from build123d import *

# Parameters (mm, degrees)
SKETCH1_W           = 35
SKETCH1_H           = 15
SKETCH1_R           = 5.5
BOSS_EXTRUDE1_DEPTH = 7
SKETCH2_W           = 4
SKETCH2_H           = 15
BOSS_EXTRUDE2_DEPTH = 40


with BuildPart() as part:
    # Sketch1 → Boss-Extrude1 (new body)
    with BuildSketch(Plane.XY):
        Rectangle(SKETCH1_W, SKETCH1_H)
        Circle(SKETCH1_R, mode=Mode.SUBTRACT)
    extrude(amount=BOSS_EXTRUDE1_DEPTH)

    # Sketch2 → Boss-Extrude2 (add)
    with BuildSketch(Plane.XY.offset(7)):
        with Locations((19.5, 0)):
            Rectangle(SKETCH2_W, SKETCH2_H)
        with Locations((-19.5, 0)):
            Rectangle(SKETCH2_W, SKETCH2_H)
    extrude(amount=-BOSS_EXTRUDE2_DEPTH)


solid = part.part
Geometry: final body of the model. Coordinates: model frame, mm. A direction names the side the tool comes from. Round coordinates to 2 decimals unless told otherwise and drop trailing zeros. Write each loop counter-clockwise with the first axis right and the second up, starting at its lowest first coordinate (ties: lowest second). Pieces come first, ordered by that corner, then holes. Notation, with made-up numbers: M 26.5,83 L 54.5,83 A14 ccw 54.5,94 Z; hole C 0.25,65.5 d8. An arc over 180 degrees is marked long. Write item = value, one per line.
Item 1: Section query C-C on y = 2. Return loops of the section in (x, z).
Findings:
outline = M -21.5,-33 L -17.5,-33 L -17.5,0 L -5.12,0 L -5.12,7 L -21.5,7 Z; M 5.12,0 L 17.5,0 L 17.5,-33 L 21.5,-33 L 21.5,7 L 5.12,7 Z
Item 2: Pull-direction query (X, two-part tool) for faces 1 (the face through (-17.5, 0, -16)), 2 (the face through (0, -7.5, 1)), 3 (the face through (-21.5, 0, -13)); classes: pulls with the +X half, pulls with the -X half, needs draft (parallel to the pull), parting line crosses it, or undercut.
Findings:
face_1 = undercut
face_2 = needs draft
face_3 = pulls with the -X half
Item 3: Material intervals for line 1 along Y through (x, z) = (0, 2); line 2 along X through (y, z) = (-2.5, -24); line 3 along Z through (x, y) = (-14.5, -0.75), sorted ascending. Write a range as [from, to].
Findings:
line_1 = [-7.5, -5.5], [5.5, 7.5]
line_2 = [-21.5, -17.5], [17.5, 21.5]
line_3 = [0, 7]
Item 4: Section query B-B on x = 0. Return loops of the section in (y, z).
Findings:
outline = M -7.5,0 L -5.5,0 L -5.5,7 L -7.5,7 Z; M 5.5,0 L 7.5,0 L 7.5,7 L 5.5,7 Z
Item 5: Access query for faces 4 (the face through (-5, 3, 7)), 5 (the face through (17.5, 0, -16)). Directions: +Z, -Z, +X, -X, +Y, -Y. A direction counts if a zero-diameter tool reaches every point of the face in a straight line with its end or side. Return the directions, or none.
Findings:
face_4 = +Z, +X, -X, +Y, -Y
face_5 = -Z, +Y, -Y
Item 6: Section query A-A on z = -18. Return loops of the section in (x, y), then the cut area to 3 significant figures.
Findings:
outline = M -21.5,-7.5 L -17.5,-7.5 L -17.5,7.5 L -21.5,7.5 Z; M 17.5,-7.5 L 21.5,-7.5 L 21.5,7.5 L 17.5,7.5 Z
area = 120 mm^2
Item 7: Pin query (flat end, axial travel): P1, Ø3, axis at x = -1, z = -2, coming from the -Y side (3 decimals); P2, Ø4.5, axis at x = 4, y = -1.5, coming from the -Z side. Return the tip coordinate at first contact, or that it passes through.
Findings:
P1 = through
P2 = 0
Item 8: Section query D-D on z = 1.5. Return loops of the section in (x, y).
Findings:
outline = M -21.5,-7.5 L 21.5,-7.5 L 21.5,7.5 L -21.5,7.5 Z; hole C 0,0 d11
